The listing builds one solid part. Answer for the finished solid, in the listing's coordinates (mm). Coordinates: 2 decimals unless noted, no trailing zeros. Write each loop counter-clockwise with the first axis right and the second up, starting at its lowest first coordinate (ties: lowest second). Pieces come first, ordered by that corner, then holes. Notation, with made-up numbers: M -5,3 L 40,3 A22 cw 40,15 Z; hole C 42,14.25 d2. An arc over 180 degrees is marked long. Answer as CSV lines item,"result".
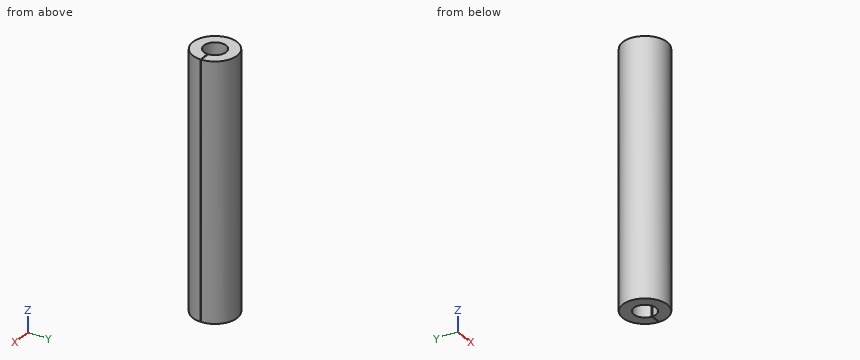
```python
from build123d import *

# Parameters (mm, degrees)
ESQUISSE1_R             = 70
BASE_EXTRUSION_DEPTH    = 800
ESQUISSE2_R             = 35
ENL_V_MAT_EXTRU_1_DEPTH = 800
ESQUISSE3_W             = 70
ESQUISSE3_H             = 2
ENL_V_MAT_EXTRU_2_DEPTH = 800


with BuildPart() as part:
    # Esquisse1 → Base-Extrusion (new body)
    with BuildSketch(Plane.XY):
        Circle(ESQUISSE1_R)
    extrude(amount=BASE_EXTRUSION_DEPTH)

    # Esquisse2 → Enlèv. mat.-Extru.1 (cut)
    with BuildSketch(Plane.XY.offset(800)):
        Circle(ESQUISSE2_R)
    extrude(amount=-ENL_V_MAT_EXTRU_1_DEPTH, mode=Mode.SUBTRACT)

    # Esquisse3 → Enlèv. mat.-Extru.2 (cut)
    with BuildSketch(Plane.XY.offset(800)):
        with Locations((45, 0)):
            Rectangle(ESQUISSE3_W, ESQUISSE3_H)
    extrude(amount=-ENL_V_MAT_EXTRU_2_DEPTH, mode=Mode.SUBTRACT)


solid = part.part
```
Q1. Flat-ended cylindrical pins translate along their axes: pin 1 Ø2 at (y, z) = (-55, 474.5) entering from -X; pin 2 Ø2 at (x, z) = (-9, 288.5) entering from +Y; pin 3 Ø12 at (x, y) = (-24, 7) entering from -Z (1 decimal). Find the tip coordinate at first contact, or state that the pin passes through.
Output:
pin 1,"x = -44.54"
pin 2,"y = 69.54"
pin 3,"through"
Q2. Find section C-C (z = 496). Give the vertices of the cut face in (x, y).
Output:
outline,"M 34.99,-1 A35 cw long 34.99,1 L 69.99,1 A70 ccw long 69.99,-1 Z"
Q3. Find section A-A (x = 0). Give the vertices of the cut face in (y, z), and give its area (3 significant figures).
Output:
outline,"M -70,0 L -35,0 L -35,800 L -70,800 Z; M 35,0 L 70,0 L 70,800 L 35,800 Z"
area,"56,000 mm2"
Q4. Straight lines are drawn through the part: line 1 (Y direction, x = 0, z = 248); line 2 (Y direction, x = 5, z = 533.5); line 3 (X direction, y = -17, z = 555.5). For each, find the intervals that lie inside material, in ascending order.
Output:
line 1,"-70 to -35, 35 to 70"
line 2,"-69.82 to -34.64, 34.64 to 69.82"
line 3,"-67.9 to -30.59, 30.59 to 67.9"
Q5. Find section B-B (y = 17). Give the vertices of the cut face in (x, z), and give its area (3 significant figures).
Output:
outline,"M -67.9,0 L -30.59,0 L -30.59,800 L -67.9,800 Z; M 30.59,0 L 67.9,0 L 67.9,800 L 30.59,800 Z"
area,"59,700 mm2"
Q6. Find section D-D (y = -59). Give the vertices of the cut face in (x, z).
Output:
outline,"M -37.67,0 L 37.67,0 L 37.67,800 L -37.67,800 Z"
